The listing builds one solid part. Answer for the finished solid, in the listing's coordinates (mm). Face numbers are marked on the shaded views. A direction names the side the tool comes from. Coordinates: 2 decimals unless noted, no trailing zeros. Order: outer loops, then holes, each group sorted by start corner. A loop starts at its lowest first (then second) coordinate and runs counter-clockwise, first axis right, second up. Notation, with made-up numbers: (1, -32.5) -> (54, -32.5) arc R6 ccw to (54, -22.5) -> close; hole circle Ø10 at (27, 30.25). An arc over 180 degrees is marked (long way). Answer in a Markdown table with one row per item.
```python
from build123d import *

# Parameters (mm, degrees)
SKETCH1_W            = 148
SKETCH1_H            = 115
BOSS_EXTRUDE4_DEPTH  = 3
SKETCH2_R            = 2.25
CUT_EXTRUDE1_DEPTH   = 3
SKETCH3_R            = 2.25
CUT_EXTRUDE2_DEPTH   = 3
SKETCH4_R            = 2.25
CUT_EXTRUDE3_DEPTH   = 3
SKETCH5_W            = 30
SKETCH5_H            = 30
BOSS_EXTRUDE7_DEPTH  = 20
SKETCH6_R            = 2.25
CUT_EXTRUDE4_DEPTH   = 10
SKETCH7_R            = 1.5
CUT_EXTRUDE5_DEPTH   = 30
SKETCH10_W           = 20
SKETCH10_H           = 51.38
CUT_EXTRUDE6_DEPTH   = 51.3
SKETCH11_W           = 20.353734706
SKETCH11_H           = 51.38
CUT_EXTRUDE7_DEPTH   = 51.3
SKETCH13_W           = 5
SKETCH13_H           = 14
CUT_EXTRUDE8_DEPTH   = 51.3
SKETCH8_W            = 3
SKETCH8_H            = 51
BOSS_EXTRUDE11_DEPTH = 53.3
SKETCH9_W            = 3
SKETCH9_H            = 51
BOSS_EXTRUDE12_DEPTH = 55.3
SKETCH15_R           = 2.25
CUT_EXTRUDE12_DEPTH  = 53.3
SKETCH14_R           = 2.25
CUT_EXTRUDE13_DEPTH  = 53.3
SKETCH17_R           = 2.25
CUT_EXTRUDE14_DEPTH  = 53.3
SKETCH18_W           = 15
SKETCH18_H           = 51.38
CUT_EXTRUDE15_DEPTH  = 10
SKETCH19_W           = 145.001760506
SKETCH19_H           = 61.096648556
BOSS_EXTRUDE13_DEPTH = 3
SKETCH20_R           = 1.5
CUT_EXTRUDE16_DEPTH  = 43
SKETCH21_W           = 109.74816289
SKETCH21_H           = 51.975747058
CUT_EXTRUDE18_DEPTH  = 43
SKETCH23_W           = 39.73104878
SKETCH23_H           = 68.636927329
CUT_EXTRUDE19_DEPTH  = 43
SKETCH24_W           = 37.931057655
SKETCH24_H           = 65.519761518
CUT_EXTRUDE20_DEPTH  = 43
SKETCH25_W           = 4
SKETCH25_H           = 12
CUT_EXTRUDE23_DEPTH  = 43


with BuildPart() as part:
    # Sketch1 → Boss-Extrude4 (new body)
    with BuildSketch(Plane(origin=(0, 0, 0), x_dir=(1, 0, 0), z_dir=(0, 1, 0))):
        with Locations((74, 57.5)):
            Rectangle(SKETCH1_W, SKETCH1_H)
    extrude(amount=BOSS_EXTRUDE4_DEPTH)

    # Sketch2 → Cut-Extrude1 (cut)
    with BuildSketch(Plane(origin=(0, 3, 0), x_dir=(1, 0, 0), z_dir=(0, 1, 0))):
        with Locations(Location((5, 110, 0), (0, 0, 270))):
            Circle(SKETCH2_R)
    extrude(amount=-CUT_EXTRUDE1_DEPTH, mode=Mode.SUBTRACT)

    # Sketch3 → Cut-Extrude2 (cut)
    with BuildSketch(Plane(origin=(0, 3, 0), x_dir=(1, 0, 0), z_dir=(0, 1, 0))):
        with Locations(Location((143, 110, 0), (0, 0, 270))):
            Circle(SKETCH3_R)
    extrude(amount=-CUT_EXTRUDE2_DEPTH, mode=Mode.SUBTRACT)

    # Sketch4 → Cut-Extrude3 (cut)
    with BuildSketch(Plane(origin=(0, 3, 0), x_dir=(1, 0, 0), z_dir=(0, 1, 0))):
        with Locations(Location((5, 56, 0), (0, 0, 270))):
            Circle(SKETCH4_R)
    extrude(amount=-CUT_EXTRUDE3_DEPTH, mode=Mode.SUBTRACT)

    # Sketch5 → Boss-Extrude7 (add)
    with BuildSketch(Plane(origin=(0, 3, 0), x_dir=(1, 0, 0), z_dir=(0, 1, 0))):
        with Locations((74, 15)):
            Rectangle(SKETCH5_W, SKETCH5_H)
    extrude(amount=BOSS_EXTRUDE7_DEPTH)

    # Sketch6 → Cut-Extrude4 (cut)
    with BuildSketch(Plane(origin=(0, 3, 0), x_dir=(1, 0, 0), z_dir=(0, 1, 0))):
        with Locations(Location((20, 110, 0), (0, 0, 270))):
            Circle(SKETCH6_R)
        with Locations(Location((35, 110, 0), (0, 0, 270))):
            Circle(SKETCH6_R)
        with Locations(Location((20, 56, 0), (0, 0, 270))):
            Circle(SKETCH6_R)
        with Locations(Location((35, 56, 0), (0, 0, 270))):
            Circle(SKETCH6_R)
        with Locations(Location((128, 110, 0), (0, 0, 270))):
            Circle(SKETCH6_R)
        with Locations(Location((113, 110, 0), (0, 0, 270))):
            Circle(SKETCH6_R)
        with Locations(Location((113, 56, 0), (0, 0, 270))):
            Circle(SKETCH6_R)
        with Locations(Location((128, 56, 0), (0, 0, 270))):
            Circle(SKETCH6_R)
        with Locations(Location((143, 56, 0), (0, 0, 270))):
            Circle(SKETCH6_R)
    extrude(amount=-CUT_EXTRUDE4_DEPTH, mode=Mode.SUBTRACT)

    # Sketch7 → Cut-Extrude5 (cut)
    with BuildSketch(Plane(origin=(0, 23, 0), x_dir=(1, 0, 0), z_dir=(0, 1, 0))):
        with Locations(Location((69.5, 20, 0), (0, 0, 270))):
            Circle(SKETCH7_R)
        with Locations(Location((74, 10, 0), (0, 0, 270))):
            Circle(SKETCH7_R)
        with Locations(Location((78.5, 20, 0), (0, 0, 270))):
            Circle(SKETCH7_R)
    extrude(amount=-CUT_EXTRUDE5_DEPTH, mode=Mode.SUBTRACT)

    # Sketch10 → Cut-Extrude6 (cut)
    with BuildSketch(Plane(origin=(0, 3, 0), x_dir=(1, 0, 0), z_dir=(0, 1, 0))):
        with Locations((138, 25.69)):
            Rectangle(SKETCH10_W, SKETCH10_H)
    extrude(amount=-CUT_EXTRUDE6_DEPTH, mode=Mode.SUBTRACT)

    # Sketch11 → Cut-Extrude7 (cut)
    with BuildSketch(Plane(origin=(0, 3, 0), x_dir=(1, 0, 0), z_dir=(0, 1, 0))):
        with Locations((9.823132647, 25.69)):
            Rectangle(SKETCH11_W, SKETCH11_H)
    extrude(amount=-CUT_EXTRUDE7_DEPTH, mode=Mode.SUBTRACT)

    # Sketch13 → Cut-Extrude8 (cut)
    with BuildSketch(Plane(origin=(0, 3, 0), x_dir=(1, 0, 0), z_dir=(0, 1, 0))):
        with Locations((27.5, 39)):
            Rectangle(SKETCH13_W, SKETCH13_H)
        with Locations((27.5, 23)):
            Rectangle(SKETCH13_W, SKETCH13_H)
        with Locations((120.5, 39)):
            Rectangle(SKETCH13_W, SKETCH13_H)
        with Locations((120.5, 23)):
            Rectangle(SKETCH13_W, SKETCH13_H)
    extrude(amount=-CUT_EXTRUDE8_DEPTH, mode=Mode.SUBTRACT)

    # Sketch8 → Boss-Extrude11 (add)
    with BuildSketch(Plane(origin=(0, 3, 0), x_dir=(1, 0, 0), z_dir=(0, 1, 0))):
        with Locations((95.5, 25.5)):
            Rectangle(SKETCH8_W, SKETCH8_H)
    extrude(amount=BOSS_EXTRUDE11_DEPTH)

    # Sketch9 → Boss-Extrude12 (add)
    with BuildSketch(Plane(origin=(0, 0, 0), x_dir=(-1, 0, 0), z_dir=(0, -1, 0))):
        with Locations((-52.5, 25.5)):
            Rectangle(SKETCH9_W, SKETCH9_H)
    extrude(amount=-BOSS_EXTRUDE12_DEPTH)

    # Sketch15 → Cut-Extrude12 (cut)
    with BuildSketch(Plane(origin=(97, 0, 0), x_dir=(0, 0, -1), z_dir=(1, 0, 0))):
        with Locations((45.4, 9.25)):
            Circle(SKETCH15_R)
    extrude(amount=-CUT_EXTRUDE12_DEPTH, mode=Mode.SUBTRACT)

    # Sketch14 → Cut-Extrude13 (cut)
    with BuildSketch(Plane(origin=(97, 0, 0), x_dir=(0, 0, -1), z_dir=(1, 0, 0))):
        with Locations((45.4, 52.25)):
            Circle(SKETCH14_R)
        with Locations((7.4, 9.25)):
            Circle(SKETCH14_R)
    extrude(amount=-CUT_EXTRUDE13_DEPTH, mode=Mode.SUBTRACT)

    # Sketch17 → Cut-Extrude14 (cut)
    with BuildSketch(Plane(origin=(97, 0, 0), x_dir=(0, 0, -1), z_dir=(1, 0, 0))):
        with Locations((7.4, 52.25)):
            Circle(SKETCH17_R)
    extrude(amount=-CUT_EXTRUDE14_DEPTH, mode=Mode.SUBTRACT)

    # Sketch18 → Cut-Extrude15 (cut)
    with BuildSketch(Plane(origin=(0, 3, 0), x_dir=(1, 0, 0), z_dir=(0, 1, 0))):
        with Locations((120.5, 25.69)):
            Rectangle(SKETCH18_W, SKETCH18_H)
        with Locations((27.5, 25.69)):
            Rectangle(SKETCH18_W, SKETCH18_H)
    extrude(amount=-CUT_EXTRUDE15_DEPTH, mode=Mode.SUBTRACT)

    # Sketch19 → Boss-Extrude13 (add)
    with BuildSketch(Plane(origin=(0, 3, 0), x_dir=(1, 0, 0), z_dir=(0, 1, 0))):
        with Locations((74.214102408, 83.006974137)):
            Rectangle(SKETCH19_W, SKETCH19_H)
    extrude(amount=-BOSS_EXTRUDE13_DEPTH)

    # Sketch20 → Cut-Extrude16 (cut)
    with BuildSketch(Plane(origin=(0, 3, 0), x_dir=(1, 0, 0), z_dir=(0, 1, 0))):
        with Locations(Location((64, 79.5, 0), (0, 0, 270))):
            Circle(SKETCH20_R)
        with Locations(Location((84, 79.5, 0), (0, 0, 270))):
            Circle(SKETCH20_R)
        with Locations(Location((64, 54.5, 0), (0, 0, 270))):
            Circle(SKETCH20_R)
        with Locations(Location((84, 54.5, 0), (0, 0, 270))):
            Circle(SKETCH20_R)
    extrude(amount=-CUT_EXTRUDE16_DEPTH, mode=Mode.SUBTRACT)

    # Sketch21 → Cut-Extrude18 (cut)
    with BuildSketch(Plane(origin=(0, 0, 0), x_dir=(-1, 0, 0), z_dir=(0, -1, 0))):
        with Locations((-79.874081445, 108.987873529)):
            Rectangle(SKETCH21_W, SKETCH21_H)
    extrude(amount=-CUT_EXTRUDE18_DEPTH, mode=Mode.SUBTRACT)

    # Sketch23 → Cut-Extrude19 (cut)
    with BuildSketch(Plane.XZ):
        with Locations((132.86552439, -85.698463665)):
            Rectangle(SKETCH23_W, SKETCH23_H)
    extrude(amount=-CUT_EXTRUDE19_DEPTH, mode=Mode.SUBTRACT)

    # Sketch24 → Cut-Extrude20 (cut)
    with BuildSketch(Plane(origin=(0, 0, 0), x_dir=(-1, 0, 0), z_dir=(0, -1, 0))):
        with Locations((-16.034471172, 84.139880759)):
            Rectangle(SKETCH24_W, SKETCH24_H)
    extrude(amount=-CUT_EXTRUDE20_DEPTH, mode=Mode.SUBTRACT)

    # Sketch25 → Cut-Extrude23 (cut)
    with BuildSketch(Plane.XZ):
        with Locations((40, -74)):
            Rectangle(SKETCH25_W, SKETCH25_H)
        with Locations((40, -60)):
            Rectangle(SKETCH25_W, SKETCH25_H)
        with Locations((108, -74)):
            Rectangle(SKETCH25_W, SKETCH25_H)
        with Locations((108, -60)):
            Rectangle(SKETCH25_W, SKETCH25_H)
    extrude(amount=-CUT_EXTRUDE23_DEPTH, mode=Mode.SUBTRACT)


solid = part.part
```
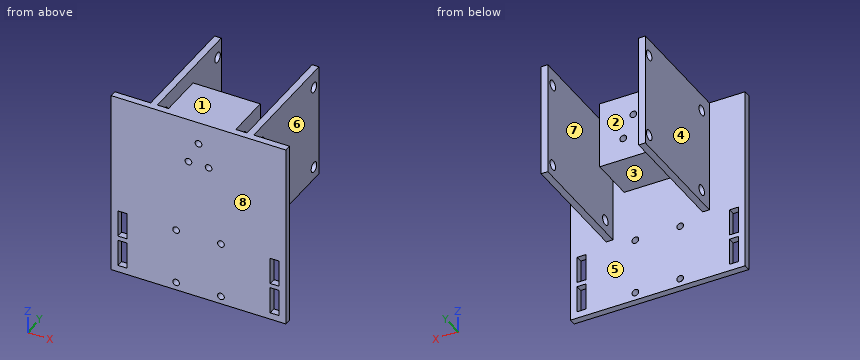
(1) A cutting plane is placed at C-C, the plane z = -71. Determine the outline of the cut face in (x, y).
Check values:
| item | result |
|---|---|
| outline | (35, 0) -> (38, 0) -> (38, 3) -> (35, 3) -> close; (42, 0) -> (106, 0) -> (106, 3) -> (42, 3) -> close; (110, 0) -> (113, 0) -> (113, 3) -> (110, 3) -> close |
(2) For a pull along X with two mould halves and no side action, classify the marked faces 5, 6, 7 and 8 as released by +X, released by -X, zero draft, split by the parting line, or undercut.
Check values:
| item | result |
|---|---|
| face 5 | undercut |
| face 6 | released by +X |
| face 7 | undercut |
| face 8 | zero draft |
(3) Which of the six approach directions +Z, -Z, +X, -X, +Y, -Y give full straight-line access (tool end or side, diameter ignored) to the marked faces 1, 2, 3 and 4?
Check values:
| item | result |
|---|---|
| face 1 | +Z, +X, -X, +Y, -Y |
| face 2 | +Z, -Z, +Y |
| face 3 | -Z, +Y |
| face 4 | +Z, -Z, -X, +Y |
(4) A cutting plane is placed at B-B, the plane x = 78.5. Determine the outline of the cut face in (y, z), then the cut area to 3 significant figures.
Check values:
| item | result |
|---|---|
| outline | (0, -83) -> (3, -83) -> (3, -30) -> (23, -30) -> (23, -21.5) -> (0, -21.5) -> close; (0, -18.5) -> (23, -18.5) -> (23, 0) -> (0, 0) -> close; hole circle Ø4.5 at (9.25, -7.4) |
| area | 764 mm² |
(5) Find the intervals of material crossed by line 1 along Y through (x, z) = (53, -7.4); line 2 along X through (y, z) = (16.25, -20); line 3 along X through (y, z) = (2.2, -79.5), in increasing order. Write a range as from..to.
Check values:
| item | result |
|---|---|
| line 1 | 0..7, 11.5..50, 54.5..55.3 |
| line 2 | 51..54, 59..68, 71..77, 80..89, 94..97 |
| line 3 | 35..38, 42..62.5, 65.5..82.5, 85.5..106, 110..113 |
(6) A cutting plane is placed at A-A, the plane y = 14. Determine the outline of the cut face in (x, z).
Check values:
| item | result |
|---|---|
| outline | (51, -51) -> (54, -51) -> (54, 0) -> (51, 0) -> close; (59, -30) -> (89, -30) -> (89, 0) -> (59, 0) -> close; (94, -51) -> (97, -51) -> (97, 0) -> (94, 0) -> close; hole circle Ø3 at (69.5, -20); hole circle Ø3 at (74, -10); hole circle Ø3 at (78.5, -20) |
(7) Flat-ended cylindrical pins translate along their axes: pin 1 (10 mm diameter, centred on x = 47, z = -23, fed in from +Y); pin 2 (5 mm diameter, centred on x = 104.5, z = -47, fed in from -Y); pin 3 (4 mm diameter, centred on x = 83.5, z = -10, fed in from +Y); pin 4 (5 mm diameter, centred on y = 52.25, z = -45.4, fed in from +X). Find the tip coordinate at first contact, or state that the pin passes through.
Check values:
| item | result |
|---|---|
| pin 1 | y = 55.3 |
| pin 2 | y = 0 |
| pin 3 | y = 23 |
| pin 4 | x = 97 |
(8) A cutting plane is placed at D-D, the plane z = -39.5. Determine the outline of the cut face in (x, y), then the cut area to 3 significant figures.
Check values:
| item | result |
|---|---|
| outline | (35, 0) -> (113, 0) -> (113, 3) -> (97, 3) -> (97, 56.3) -> (94, 56.3) -> (94, 3) -> (54, 3) -> (54, 55.3) -> (51, 55.3) -> (51, 3) -> (35, 3) -> close |
| area | 551 mm² |
